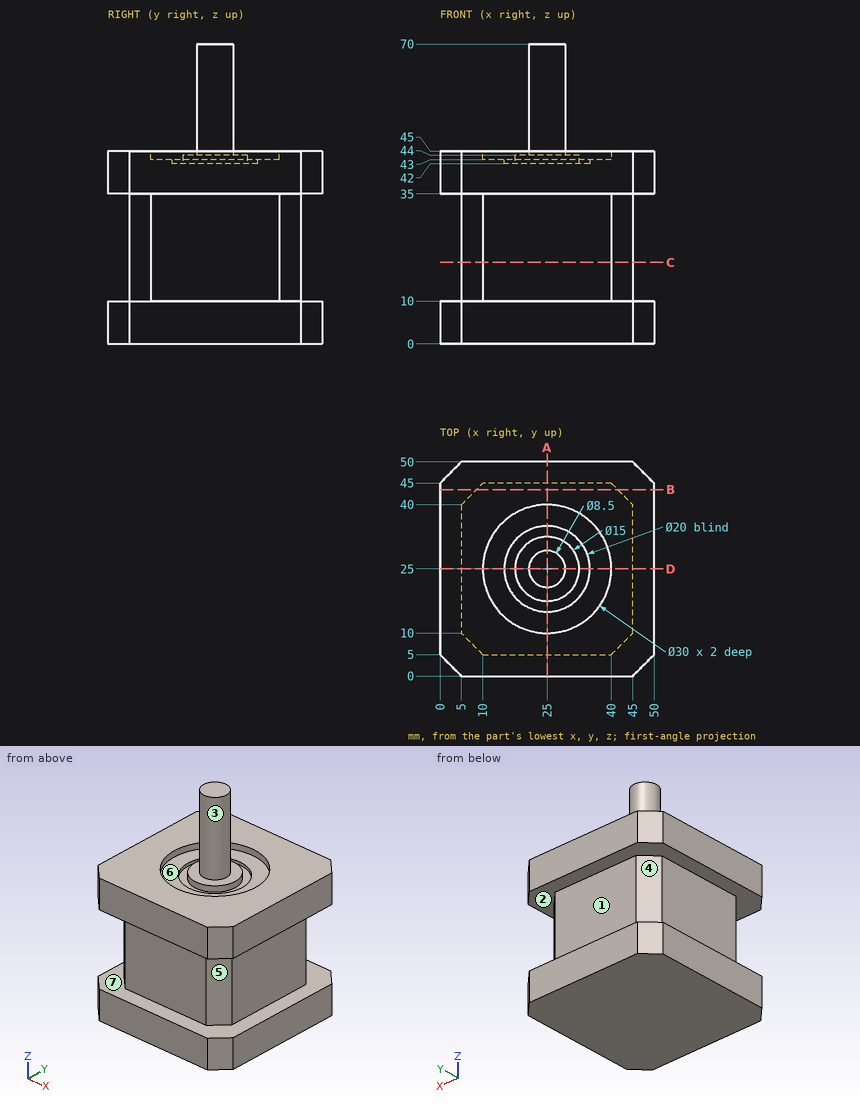
Part print with two shaded views. Sizes in mm from the minimum x, y, z corner. A direction names the side the tool comes from. Coordinates: 2 decimals unless noted, no trailing zeros. Write each loop counter-clockwise with the first axis right and the second up, starting at its lowest first coordinate (ties: lowest second). Pieces come first, ordered by that corner, then holes.
1. Drill centre lines: probe 1 along Y at (x, z) = (25, 43.45); probe 2 along Y at (x, z) = (25, 42.75); probe 3 along Z at (x, y) = (3, 27). Where is each one in solid material? Low to high.
Answer block:
probe 1: y = 0 to 10, 17.5 to 32.5, 40 to 50
probe 2: y = 0 to 15, 17.5 to 32.5, 35 to 50
probe 3: z = 0 to 10, 35 to 45
2. Band-saw the part on A-A, the plane x = 25. Give the cut face in (y, z).
Answer block:
outline: (0, 0) - (50, 0) - (50, 10) - (45, 10) - (45, 35) - (50, 35) - (50, 45) - (40, 45) - (40, 43) - (35, 43) - (35, 42) - (32.5, 42) - (32.5, 44) - (29.25, 44) - (29.25, 70) - (20.75, 70) - (20.75, 44) - (17.5, 44) - (17.5, 42) - (15, 42) - (15, 43) - (10, 43) - (10, 45) - (0, 45) - (0, 35) - (5, 35) - (5, 10) - (0, 10) - close
3. Band-saw the part on B-B, the plane y = 43.5. Give the cut face in (x, z).
Answer block:
outline: (0, 0) - (50, 0) - (50, 10) - (41.5, 10) - (41.5, 35) - (50, 35) - (50, 45) - (0, 45) - (0, 35) - (8.5, 35) - (8.5, 10) - (0, 10) - close
4. 3-axis set-ups, long thin cutter, end or side, ignore diameter. For the marked faces 1, 2 and 3: which of +Z, -Z, +X, -X, +Y, -Y reach the whole face in a straight line?
Answer block:
face 1: +X, -X, +Y
face 2: none
face 3: +Z
5. Band-saw the part on C-C, the plane z = 19. Give the cut face in (x, y), and give its area (3 significant figures).
Answer block:
outline: (5, 10) - (10, 5) - (40, 5) - (45, 10) - (45, 40) - (40, 45) - (10, 45) - (5, 40) - close
area: 1,550 mm2
6. Pull direction Y, two halves, no side cores. Call the marked faces 4, 5, 6 and 7: released by +Y, released by -Y, zero draft, split by the parting line, or undercut.
Answer block:
face 4: released by +Y
face 5: released by -Y
face 6: undercut
face 7: zero draft
7. Drop flat-ended pins along their axis: pin 1 (8 mm diameter, centred on y = 21.5, z = 23, fed in from +X); pin 2 (12.5 mm diameter, centred on x = 25.5, z = 23, fed in from +Y); pin 3 (3 mm diameter, centred on y = 7.5, z = 28.5, fed in from +X). Give the stop position or say it passes through.
Answer block:
pin 1: stops at x = 45
pin 2: stops at y = 45
pin 3: stops at x = 44
